Geometry check sheet. Reference: the model listing, model coordinates, mm. Face numbers are marked on the shaded views. A direction names the side the tool comes from. Round coordinates to 2 decimals unless told otherwise and drop trailing zeros. Order: outer loops, then holes, each group sorted by start corner. A loop starts at its lowest first (then second) coordinate and runs counter-clockwise, first axis right, second up. Notation, with made-up numbers: (13, 17.5) - (20, 17.5) arc R21 ccw to (20, 56.5) - close; hole circle Ø2 at (64.5, 28). An arc over 180 degrees is marked (long way). Return JSON: item names as keys, results as strings. Group by question number.
Q1. Sectioned sample at B-B, the plane z = 0. Record the cut outline in (x, y) (3 decimals).
Q2. Sectioned sample at A-A, the plane x = 0. Record the cut outline in (y, z) (3 decimals).
Q3. Material ranges on line 1 along Z through (x, y) = (0, -6.75); line 2 along Y through (x, z) = (-1.75, -3.5); line 3 along Y through (x, z) = (0, -7.75), recorded low to high.
Q4. Tool access check on the marked faces 4 and 5. Record the directions out of +Z, -Z, +X, -X, +Y, -Y that give a thin tool (end or side, any length) a straight path to the whole face; none if there is none.
Q5. Gauge pin test, flat ends, axial feed: pin 1 Ø10 at (x, z) = (0, 0) entering from -Y; pin 2 Ø3 at (x, z) = (0, 0.5) entering from -Y; pin 3 Ø4 at (y, z) = (0, -6) entering from -X; pin 4 Ø6 at (y, z) = (-3, -0.5) entering from +X. Record the tip position at first contact, or that the pin passes through.
Q6. Sectioned sample at C-C, the plane y = 0.75. Record the cut outline in (x, z) (3 decimals).
Q7. Sectioned sample at D-D, the plane y = 3.25. Record the cut outline in (x, z) (3 decimals), then the cut area to 3 significant figures.
Q8. Draft check along Z on the marked faces 1, 2 and 3. Enter one of: pulls with the +Z half, pulls with the -Z half, needs draft (parallel to the pull), parting line crosses it, or undercut.
```python
from build123d import *

# Parameters (mm, degrees)
SKETCH2_R          = 3.175
CUT_EXTRUDE1_DEPTH = 7
CUT_EXTRUDE2_REACH = 11.5
SKETCH3_R          = 1.1303


with BuildPart() as part:
    # Sketch1 → Revolve1 (revolve)
    with BuildSketch(Plane.XY):
        Polygon((0, 8.5), (8.5, 8.5), (9.5, 7.5), (9.5, -8.5), (8.5, -8.5), (8.5, -3.5), (5.5, -0.5), (0, -0.5), align=None)
    revolve(axis=Axis((0, 8.5, 0), (0, -1, 0)))

    # Sketch2 → Cut-Extrude1 (cut)
    with BuildSketch(Plane.XZ.offset(0.5)):
        Circle(SKETCH2_R)
    extrude(amount=-CUT_EXTRUDE1_DEPTH, mode=Mode.SUBTRACT)

    # Sketch3 → Cut-Extrude2 (cut, up to next)
    with BuildSketch(Plane.XY, mode=Mode.PRIVATE) as cut_extrude2_sk1:
        with Locations((0, 2.5)):
            Circle(SKETCH3_R)
    cut_extrude2_tool1 = extrude(cut_extrude2_sk1.sketch, amount=-CUT_EXTRUDE2_REACH, mode=Mode.PRIVATE) & part.part
    add(cut_extrude2_tool1.solids().sort_by_distance((0, 2.5, 0))[0], mode=Mode.SUBTRACT)


solid = part.part
```
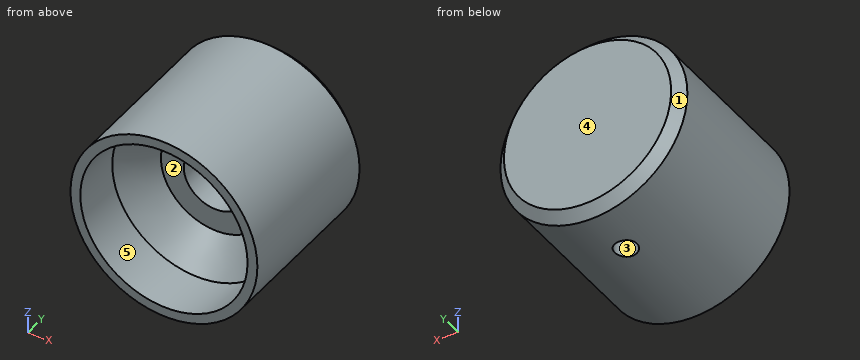
Reply:
{
 "1": {"outline": "(-9.5, -8.5) - (-8.5, -8.5) - (-8.5, -3.5) - (-5.5, -0.5) - (-3.175, -0.5) - (-3.175, 6.5) - (3.175, 6.5) - (3.175, -0.5) - (5.5, -0.5) - (8.5, -3.5) - (8.5, -8.5) - (9.5, -8.5) - (9.5, 7.5) - (8.5, 8.5) - (-8.5, 8.5) - (-9.5, 7.5) - close"},
 "2": {"outline": "(-8.5, -9.5) - (1.37, -9.5) - (1.37, -3.175) - (-0.5, -3.175) - (-0.5, -5.5) - (-3.5, -8.5) - (-8.5, -8.5) - close; (-8.5, 8.5) - (-3.5, 8.5) - (-0.5, 5.5) - (-0.5, 3.175) - (6.5, 3.175) - (6.5, -3.175) - (3.63, -3.175) - (3.63, -9.5) - (7.5, -9.5) - (8.5, -8.5) - (8.5, 8.5) - (7.5, 9.5) - (-8.5, 9.5) - close"},
 "3": {"line 1": "-9.5 to -8.5, 8.5 to 9.5", "line 2": "-0.5 to 8.5", "line 3": "-2.75 to 1.37, 3.63 to 8.5"},
 "4": {"face 4": "+Z, -Z, +X, -X, +Y", "face 5": "-Y"},
 "5": {"pin 1": "y = -0.5", "pin 2": "y = 6.5", "pin 3": "x = -8.62", "pin 4": "x = 9.5"},
 "6": {"outline": "circle Ø19 at (0, 0); hole circle Ø6.35 at (0, 0)"},
 "7": {"outline": "(-0.846, -9.462) - (-0.846, -3.06) arc R3.175 cw (long way) to (0.846, -3.06) - (0.846, -9.462) arc R9.5 ccw (long way) to start", "area": "241 mm^2"},
 "8": {"face 1": "parting line crosses it", "face 2": "undercut", "face 3": "needs draft"}
}
